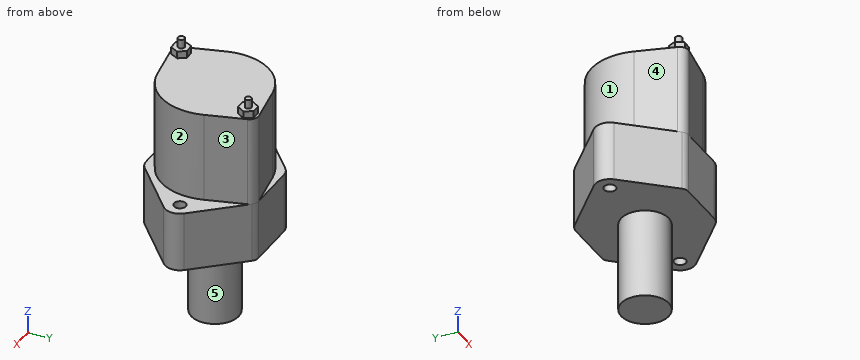
```python
from build123d import *

# Parameters (mm, degrees)
SKETCH_1_R      = 1
EXTRUDE_1_DEPTH = 10
EXTRUDE_2_DEPTH = 15
SKETCH_3_R      = 4
EXTRUDE_3_DEPTH = 15
FILLET_1_R      = 1.5
FILLET_2_R      = 2.5
EXTRUDE_4_DEPTH = 1.2
SKETCH_9_R      = 0.527306968
EXTRUDE_5_DEPTH = 1.5
SKETCH_10_R     = 0.558325025
EXTRUDE_6_DEPTH = 1.5


with BuildPart() as part:
    # Эскиз1 → Вытянуть1 (new body)
    with BuildSketch(Plane.XY):
        with BuildLine():
            Line((9.501316689, 7.607009807), (19.501316689, 7.607009807))
            Line((19.501316689, 7.607009807), (28.660908483, 15.737315961))
            ThreePointArc((28.660908483, 15.737315961), (29.496729836, 17.455638669), (28.874738709, 19.262391918))
            Line((28.874738709, 19.262391918), (21.501316689, 27.607009807))
            Line((21.501316689, 27.607009807), (11.501316689, 27.607009807))
            Line((11.501316689, 27.607009807), (2.341724894, 19.476703653))
            ThreePointArc((2.341724894, 19.476703653), (1.505903541, 17.758380944), (2.127894668, 15.951627696))
            Line((2.127894668, 15.951627696), (9.501316689, 7.607009807))
        make_face()
        with Locations(Location((27.001316689, 17.607009807, 0), (0, 0, 180))):
            Circle(SKETCH_1_R, mode=Mode.SUBTRACT)
        with Locations(Location((4.001316689, 17.607009807, 0), (0, 0, 180))):
            Circle(SKETCH_1_R, mode=Mode.SUBTRACT)
    extrude(amount=EXTRUDE_1_DEPTH)

    # Эскиз2 → Вытянуть2 (add)
    with BuildSketch(Plane.XY.offset(10)):
        with BuildLine():
            Line((22.264471235, 26.529000138), (24.137824651, 20.138951792))
            ThreePointArc((24.137824651, 20.138951792), (23.128766256, 12.82977074), (16.993089347, 8.73150338))
            Line((16.993089347, 8.73150338), (10.426208912, 7.627758736))
            ThreePointArc((10.426208912, 7.627758736), (9.381373625, 7.835768212), (8.738162142, 8.685019476))
            Line((8.738162142, 8.685019476), (6.864808726, 15.075067822))
            ThreePointArc((6.864808726, 15.075067822), (7.873867121, 22.384248873), (14.00954403, 26.482516234))
            Line((14.00954403, 26.482516234), (20.576424465, 27.586260878))
            ThreePointArc((20.576424465, 27.586260878), (21.621259753, 27.378251401), (22.264471235, 26.529000138))
        make_face()
    extrude(amount=EXTRUDE_2_DEPTH)

    # Эскиз3 → Вытянуть3 (add)
    with BuildSketch(Plane(origin=(0, 0, 0), x_dir=(-1, 0, 0), z_dir=(0, 0, -1))):
        with Locations(Location((-15.501316689, 17.607009807, 0), (0, 0, 180))):
            Circle(SKETCH_3_R)
    extrude(amount=EXTRUDE_3_DEPTH)

    # Скругление1
    fillet_1_edges = [part.edges().sort_by_distance(p)[0] for p in [
        (9.501316689, 7.607009807, 5),
        (21.501316689, 27.607009807, 5),
    ]]
    fillet(fillet_1_edges, radius=FILLET_1_R - 0.0001)  # a hair under: the kernel refuses the full size

    # Скругление2
    fillet_2_edges = [part.edges().sort_by_distance(p)[0] for p in [
        (19.501316689, 7.607009807, 5),
        (11.501316689, 27.607009807, 5),
    ]]
    fillet(fillet_2_edges, radius=FILLET_2_R)

    # Эскиз8 → Вытянуть4 (add)
    with BuildSketch(Plane.XY.offset(25)):
        Polygon((20.046142028, 27.162033609), (19.274705601, 25.87537183), (20.003269175, 24.563957398), (21.503269175, 24.539204745), (22.274705601, 25.825866524), (21.546142028, 27.137280956), align=None)
        Polygon((11.07675483, 10.680633722), (9.57675483, 10.59059908), (8.904727117, 9.246543654), (9.732699404, 7.992522869), (11.232699404, 8.082557511), (11.904727117, 9.426612937), align=None)
    extrude(amount=EXTRUDE_4_DEPTH)

    # Эскиз9 → Вытянуть5 (add)
    with BuildSketch(Plane.XY.offset(26.2)):
        with Locations(Location((20.820913454, 25.904340038, 0), (0, 0, 180))):
            Circle(SKETCH_9_R)
    extrude(amount=EXTRUDE_5_DEPTH)

    # Эскиз10 → Вытянуть6 (add)
    with BuildSketch(Plane.XY.offset(26.2)):
        with Locations(Location((10.367828265, 9.340697632, 0), (0, 0, 180))):
            Circle(SKETCH_10_R)
    extrude(amount=EXTRUDE_6_DEPTH)


solid = part.part
```
For this review, take the finished solid that the model builds, in its own axes (mm). Face numbers are marked on the shaded views. A direction names the side the tool comes from. Coordinates: 2 decimals unless noted, no trailing zeros. Order: outer loops, then holes, each group sorted by start corner. A loop starts at its lowest first (then second) coordinate and runs counter-clockwise, first axis right, second up. Notation, with made-up numbers: (24.25, 37.25) -> (77.25, 37.25) arc R20 cw to (77.25, 72.25) -> close; hole circle Ø11 at (-27, -29.75). An arc over 180 degrees is marked (long way). Use CSV: the item, a comma, the result in double quotes. Start each with the question number.
Item 1: Insertion check: pin 1 (6 mm diameter, centred on x = 11, z = 15.5, fed in from -Y); pin 2 (1 mm diameter, centred on x = 7.5, y = 23, fed in from +Z); pin 3 (2 mm diameter, centred on x = 10.5, y = 25.5, fed in from -Z); pin 4 (10 mm diameter, centred on x = 6, y = 15, fed in from +Z). Each pin has a flat end and moves straight along its axis. Give the tip position at first contact, or say it passes through.
Item 2: We need section B-B, the plane y = 23.25. Give the boundary of the cut face in (x, z), then the cut area to 3 significant figures.
Item 3: We need section A-A, the plane z = 6. Give the boundary of the cut face in (x, y).
Item 4: Wall thickness on probe 1 along X at (y, z) = (17.5, 8); probe 2 along Z at (x, y) = (11, 11); probe 3 along X at (y, z) = (17.5, -11): over which ranges is each line inside the solid? List them lowest first.
Item 5: We need section D-D, the plane z = -6. Give the boundary of the cut face in (x, y).
Item 6: We need section C-C, the plane x = 7.5. Give the boundary of the cut face in (y, z).
Item 7: For the marked faces 1, 2, 3, 4 and 5, list the 3-axis set-ups (+Z, -Z, +X, -X, +Y, -Y) from which the entire face can be reached by the end or side of a thin tool; tool diameter is ignored.
Derived:
1,pin 1,"stops at y = 7.61"
1,pin 2,"stops at z = 10"
1,pin 3,"stops at z = 0"
1,pin 4,"stops at z = 25"
2,outline,"(6.59, 0) -> (25.35, 0) -> (25.35, 10) -> (23.23, 10) -> (23.23, 25) -> (8.49, 25) -> (8.49, 10) -> (6.59, 10) -> close"
2,area,"409 mm^2"
3,outline,"(2.13, 15.95) -> (9.05, 8.11) arc R1.5 ccw to (10.18, 7.61) -> (18.55, 7.61) arc R2.5 ccw to (20.21, 8.24) -> (28.66, 15.74) arc R2.5 ccw to (28.87, 19.26) -> (21.95, 27.1) arc R1.5 ccw to (20.83, 27.61) -> (12.45, 27.61) arc R2.5 ccw to (10.79, 26.98) -> (2.34, 19.48) arc R2.5 ccw to start; hole circle Ø2 at (4, 17.61); hole circle Ø2 at (27, 17.61)"
4,probe 1,"x = 1.5 to 3.01, 5 to 26.01, 28 to 29.5"
4,probe 2,"z = 0 to 25"
4,probe 3,"x = 11.5 to 19.5"
5,outline,"circle Ø8 at (15.5, 17.61)"
6,outline,"(9.87, 0) -> (24.06, 0) -> (24.06, 10) -> (21.73, 10) -> (21.73, 25) -> (12.91, 25) -> (12.91, 10) -> (9.87, 10) -> close"
7,face 1,"+Z, -X"
7,face 2,"+Z, +X"
7,face 3,"+Z, +X, +Y"
7,face 4,"+Z, -X, -Y"
7,face 5,"-Z"
